```python
from build123d import *

# Parameters (mm, degrees)
F1_DEPTH       = 13
F2_T1_DEPTH    = 13
F4_D           = 3.3
F4_CBORE_D     = 6.5
F4_CBORE_DEPTH = 1.5


# Not quite as in the source:
# - a fillet or chamfer that OpenCascade refuses, or shapes differently, is made with other operations: its cross-section is extruded or revolved along the edge and cut away or added


with BuildPart() as f1:
    # F0 (on Top) → F1 (new body)
    with BuildSketch(Plane.XY):
        with BuildLine():
            Line((6.184642151, 5.8486273885), (-0.815357849, 5.8486273885))
            Line((-0.815357849, 5.8486273885), (-0.815357849, -29.1513726115))
            Line((-0.815357849, -29.1513726115), (3.1407309243, -29.1513726115))
            Line((3.1407309243, -29.1513726115), (3.1407309243, -4.0674617201))
            Line((3.1407309243, -4.0674617201), (7.0968196975, -4.0674617201))
            ThreePointArc((7.0968196975, -4.0674617201), (11.1636202361, 1.3066418299), (6.184642151, 5.8486273885))
        make_face()
    extrude(amount=F1_DEPTH)

    # F2: fillet of radius 5 on 1 edges, made by hand

    # F2_s2 → F2_t1 (join)
    with BuildSketch(Plane.XY):
        with BuildLine():
            ThreePointArc((7.0968196975, -4.0674617201), (4.2536011262, -5.8124001647), (3.1407309243, -8.9572724885))
            Line((3.1407309243, -8.9572724885), (3.1407309243, -4.0674617201))
            Line((3.1407309243, -4.0674617201), (7.0968196975, -4.0674617201))
        make_face()
    extrude(amount=F2_T1_DEPTH)

    # F4 (through all)
    with Locations(Plane.YZ.offset(3.1407309243)):
        with Locations((-22.1513726115, 6.5), (-14.1513726115, 6.5)):
            CounterBoreHole(F4_D / 2, F4_CBORE_D / 2, F4_CBORE_DEPTH)


solid = f1.part
```
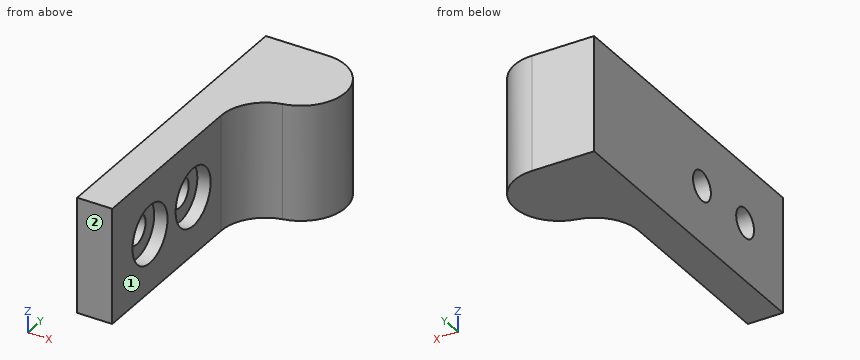
Source: CAD feature listing. Evaluate the final solid. Frame: model axes, mm. Face numbers are marked on the shaded views. A direction names the side the tool comes from. Round coordinates to 2 decimals unless told otherwise and drop trailing zeros. Order: outer loops, then holes, each group sorted by start corner. A loop starts at its lowest first (then second) coordinate and runs counter-clockwise, first axis right, second up. Notation, with made-up numbers: (-35, 3.5) -> (-22, 3.5) arc R18 ccw to (-22, 19.5) -> close; hole circle Ø4 at (-24, 1). An arc over 180 degrees is marked (long way). One line per item, written item: value. Start each with the question number.
Q1. Section query C-C (z = 3.75). Return the cut outline in (x, y), plus the area to 3 significant figures.
Q2. Section query A-A (z = 6.5). Return the cut outline in (x, y), plus the area to 3 significant figures.
Q3. Material intervals for probe 1 along X at (y, z) = (-26, 9.5); probe 2 along X at (y, z) = (-12.5, 8); probe 3 along Z at (x, y) = (0, -21), sorted ascending.
Q4. Access query for the marked faces 1 and 2. Directions: +Z, -Z, +X, -X, +Y, -Y. A direction counts if a zero-diameter tool reaches every point of the face in a straight line with its end or side. Return the directions, or none.
Q5. Section query D-D (x = 10). Return the cut outline in (y, z), plus the area to 3 significant figures.
Q6. Section query B-B (y = -11.5). Return the cut outline in (x, z), plus the area to 3 significant figures.
Q7. Pin query (flat end, axial travel): pin 1 (4 mm diameter, centred on x = 5.5, y = -2, fed in from -Z); pin 2 (2 mm diameter, centred on y = -14.15, z = 6.5, fed in from -X); pin 3 (1.5 mm diameter, centred on x = 6.5, z = 5, fed in from -Y); pin 4 (5 mm diameter, centred on y = -13.5, z = 7.5, fed in from +X). Return the tip coordinate at first contact, or that it passes through.
Findings below:
1. outline: (-0.82, -29.15) -> (3.14, -29.15) -> (3.14, -23.88) -> (1.64, -23.88) -> (1.64, -20.42) -> (3.14, -20.42) -> (3.14, -15.88) -> (1.64, -15.88) -> (1.64, -12.42) -> (3.14, -12.42) -> (3.14, -8.96) arc R5 cw to (7.1, -4.07) arc R5 ccw to (6.18, 5.85) -> (-0.82, 5.85) -> close
1. area: 202 mm²
2. outline: (-0.82, -29.15) -> (3.14, -29.15) -> (3.14, -25.4) -> (1.64, -25.4) -> (1.64, -23.8) -> (-0.82, -23.8) -> close; (-0.82, -20.5) -> (1.64, -20.5) -> (1.64, -18.9) -> (3.14, -18.9) -> (3.14, -17.4) -> (1.64, -17.4) -> (1.64, -15.8) -> (-0.82, -15.8) -> close; (-0.82, -12.5) -> (1.64, -12.5) -> (1.64, -10.9) -> (3.14, -10.9) -> (3.14, -8.96) arc R5 cw to (7.1, -4.07) arc R5 ccw to (6.18, 5.85) -> (-0.82, 5.85) -> close
2. area: 177 mm²
3. probe 1: -0.82 to 3.14
3. probe 2: -0.82 to 1.64
3. probe 3: 0 to 5.32, 7.68 to 13
4. face 1: +Z, -Z, +X, -Y
4. face 2: +Z, -Z, +X, -X, -Y
5. outline: (-2.38, 0) -> (4.08, 0) -> (4.08, 13) -> (-2.38, 13) -> close
5. area: 84.0 mm²
6. outline: (-0.82, 0) -> (3.14, 0) -> (3.14, 4.62) -> (1.64, 4.62) -> (1.64, 8.38) -> (3.14, 8.38) -> (3.14, 13) -> (-0.82, 13) -> close
6. area: 45.8 mm²
7. pin 1: z = 0
7. pin 2: through
7. pin 3: y = -4.57
7. pin 4: x = 3.14
